Here's how the part is built. I have some questions about the finished solid (model axes, mm). Face numbers are marked on the shaded views. A direction names the side the tool comes from. Round coordinates to 2 decimals unless told otherwise and drop trailing zeros. Write each loop counter-clockwise with the first axis right and the second up, starting at its lowest first coordinate (ties: lowest second). Pieces come first, ordered by that corner, then holes. Notation, with made-up numbers: (38, -30.75) - (93, -30.75) arc R19 ccw to (93, -12.75) - close; hole circle Ø9 at (83.25, 38). An arc over 180 degrees is marked (long way). One line per question, with ' | ' between items. Start each with the question number.
(1) Will these pins go through, and if not, where does the flat tip stop? pin 1 (4 mm diameter, centred on x = 3, y = 5, fed in from -Z); pin 2 (1.5 mm diameter, centred on x = -4.5, z = 11.5, fed in from +Y); pin 3 (6 mm diameter, centred on x = -4.5, z = 6, fed in from -Y).
(2) Thinking about a two-plate mould opening in Y: for the marked faces 4, 5 and 6, which applies, pulls with the +Y half, pulls with the -Y half, needs draft (parallel to the pull), parting line crosses it, or undercut?
(3) If I drill on L1, parallel to Y at x = 0, z = 9.5; L2, parallel to X at y = -0.5, z = 14.5; L3, parallel to Y at x = 0, z = 21.05, over which ranges is the centre line in solid material (lowest first)?
(4) Imagine slicing it at A-A (x = 0). Write out the boundary of the cut face in (y, z), plus the area to 4 significant figures.
(5) For the marked faces 1, 2 and 3, which set-ups out of +Z, -Z, +X, -X, +Y, -Y let a thin tool reach every point of the face, with its end or its side?
(6) Imagine slicing it at C-C (y = -11.5). Write out the boundary of the cut face in (x, z).
(7) Imagine slicing it at D-D (x = -15). Write out the boundary of the cut face in (y, z).
from build123d import *

# Parameters (mm, degrees)
F0_R     = 30
F1_DEPTH = 2
F2_R     = 25.75
F3_DEPTH = 21
F4_R     = 20
F5_DEPTH = 18
F6_R     = 3
F7_DEPTH = 5.001


with BuildPart() as f1:
    # F0 (on Top) → F1 (new body)
    with BuildSketch(Plane.XY):
        Circle(F0_R)
    extrude(amount=F1_DEPTH)

    # F2 (on face) → F3 (join)
    with BuildSketch(Plane.XY.offset(2)):
        Circle(F2_R)
    extrude(amount=F3_DEPTH)

    # F4 (on face) → F5 (cut)
    with BuildSketch(Plane(origin=(0, 0, 0), x_dir=(1, 0, 0), z_dir=(0, 0, -1))):
        Circle(F4_R)
    extrude(amount=-F5_DEPTH, mode=Mode.SUBTRACT)

    # F6 (on face) → F7 (cut, through all)
    with BuildSketch(Plane(origin=(0, 0, 18), x_dir=(1, 0, 0), z_dir=(0, 0, -1))):
        Circle(F6_R)
    extrude(amount=-F7_DEPTH, mode=Mode.SUBTRACT)


solid = f1.part
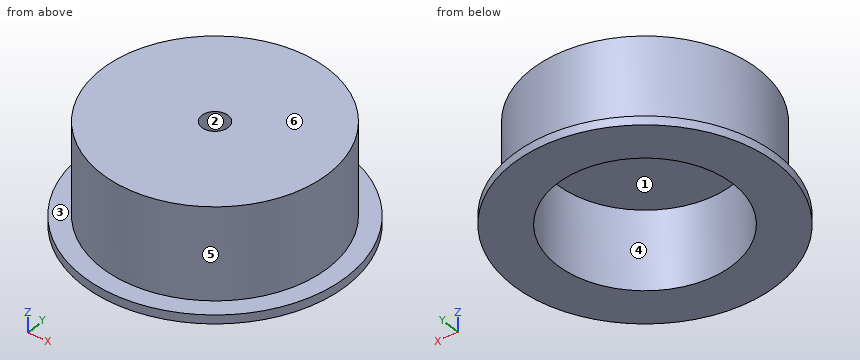
Check sheet entries:
1) pin 1: z = 18 | pin 2: y = 25.48 | pin 3: y = -25.71
2) face 4: undercut | face 5: parting line crosses it | face 6: needs draft
3) L1: -25.75 to -20, 20 to 25.75 | L2: -25.75 to -19.99, 19.99 to 25.75 | L3: -25.75 to -3, 3 to 25.75
4) outline: (-30, 0) - (-20, 0) - (-20, 18) - (-3, 18) - (-3, 23) - (-25.75, 23) - (-25.75, 2) - (-30, 2) - close; (3, 18) - (20, 18) - (20, 0) - (30, 0) - (30, 2) - (25.75, 2) - (25.75, 23) - (3, 23) - close | area: 451.5 mm^2
5) face 1: -Z | face 2: +Z, -Z | face 3: +Z
6) outline: (-27.71, 0) - (-16.36, 0) - (-16.36, 18) - (16.36, 18) - (16.36, 0) - (27.71, 0) - (27.71, 2) - (23.04, 2) - (23.04, 23) - (-23.04, 23) - (-23.04, 2) - (-27.71, 2) - close
7) outline: (-25.98, 0) - (-13.23, 0) - (-13.23, 18) - (13.23, 18) - (13.23, 0) - (25.98, 0) - (25.98, 2) - (20.93, 2) - (20.93, 23) - (-20.93, 23) - (-20.93, 2) - (-25.98, 2) - close
